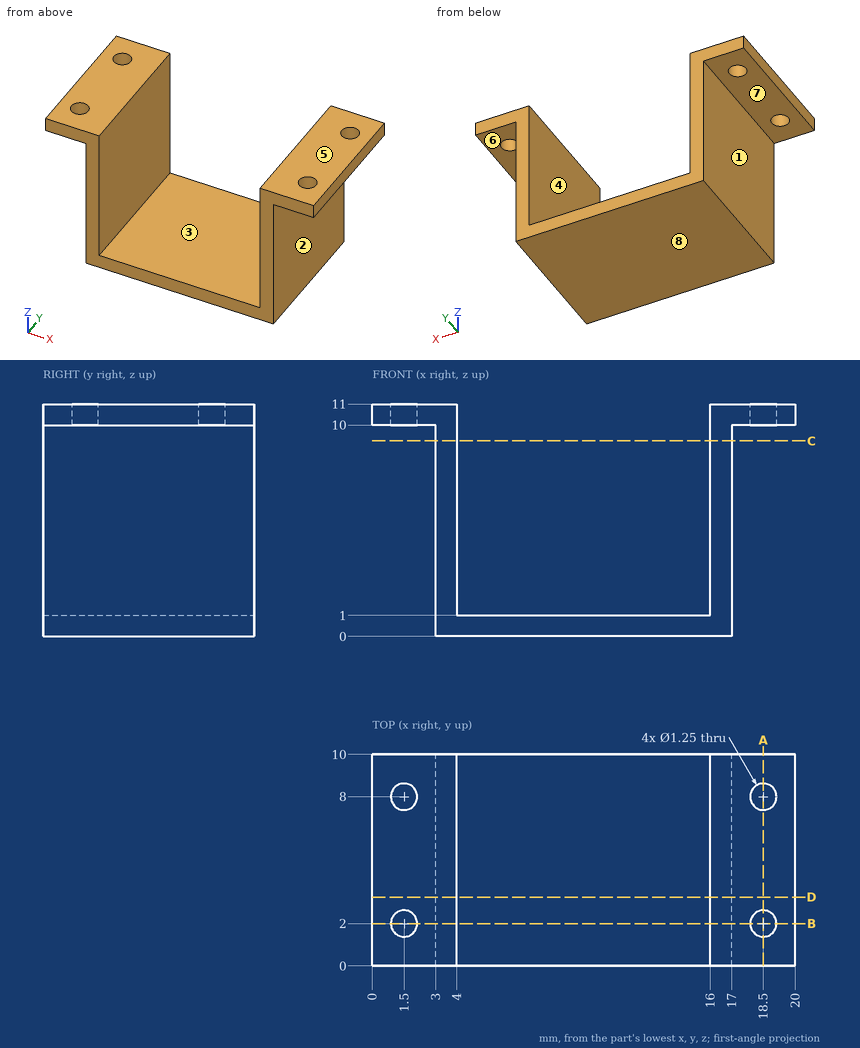
Can you work these out from the drawing? Everything is in mm from the part's minimum corner. A direction names the side the tool comes from. Coordinates: 2 decimals unless noted, no trailing zeros. Order: outer loops, then holes, each group sorted by start corner. A loop starts at its lowest first (then second) coordinate and runs counter-clockwise, first axis right, second up. Notation, with made-up numbers: M -27,54 L 30,54 A15 cw 30,61 Z; hole C 79.5,21 d3. An arc over 180 degrees is marked long. Answer as CSV lines item,"result". Start each with the question number.
1. For pin 1 (1.1 mm diameter, centred on x = 18.5, y = 2, fed in from -Z); pin 2 (3.5 mm diameter, centred on x = 1, y = 6, fed in from -Z); pin 3 (4 mm diameter, centred on x = 5, z = 6.5, fed in from +Y); pin 4 (3 mm diameter, centred on y = 3.5, z = 6, fed in from +X), each with a flat end and sliding along its axis, tell me the tip position at first contact or that it passes through.
2. I want a section at C-C, the plane z = 9.25. Write out the boundary of the cut face in (x, y), and give its area (3 significant figures).
3. I want a section at A-A, the plane x = 18.5. Write out the boundary of the cut face in (y, z) (3 decimals), and give its area (3 significant figures).
4. On a 3-axis mill with a long thin cutter (end or side, diameter ignored), from which of +Z, -Z, +X, -X, +Y, -Y can I reach the whole of each face in a straight line? I mean the marked faces 4, 5, 6, 7 and 8. Say none if no direction works.
5. We'd pull the mould along X, two halves only. Please class the marked faces 1, 2 and 3: released by +X, released by -X, zero draft, split by the parting line, or undercut.
6. I need wall thicknesses on line 1 (Y direction, x = 1.5, z = 10.65) (3 decimals); line 2 (X direction, y = 8.5, z = 7.25); line 3 (Z direction, x = 11, y = 2). Which ranges of each line are inside material? Lowest first, please. Write a range as [from, to].
7. I want a section at B-B, the plane y = 2. Write out the boundary of the cut face in (x, z) (3 decimals), and give its area (3 significant figures).
8. I want a section at D-D, the plane y = 3.25. Write out the boundary of the cut face in (x, z), and give its area (3 significant figures).
Recorded:
1,pin 1,"passes through"
1,pin 2,"stops at z = 10"
1,pin 3,"stops at y = 10"
1,pin 4,"stops at x = 17"
2,outline,"M 3,0 L 4,0 L 4,10 L 3,10 Z; M 16,0 L 17,0 L 17,10 L 16,10 Z"
2,area,"20.0 mm2"
3,outline,"M 0,10 L 1.375,10 L 1.375,11 L 0,11 Z; M 2.625,10 L 7.375,10 L 7.375,11 L 2.625,11 Z; M 8.625,10 L 10,10 L 10,11 L 8.625,11 Z"
3,area,"7.50 mm2"
4,face 4,"+Z, +Y, -Y"
4,face 5,"+Z, +X, -X, +Y, -Y"
4,face 6,"-Z, +X, +Y, -Y"
4,face 7,"-Z, -X, +Y, -Y"
4,face 8,"-Z, +X, -X, +Y, -Y"
5,face 1,"released by -X"
5,face 2,"released by +X"
5,face 3,"undercut"
6,line 1,"y = [0, 1.375], [2.625, 7.375], [8.625, 10]"
6,line 2,"x = [3, 4], [16, 17]"
6,line 3,"z = [0, 1]"
7,outline,"M 0,10 L 0.875,10 L 0.875,11 L 0,11 Z; M 2.125,10 L 3,10 L 3,0 L 17,0 L 17,10 L 17.875,10 L 17.875,11 L 16,11 L 16,1 L 4,1 L 4,11 L 2.125,11 Z; M 19.125,10 L 20,10 L 20,11 L 19.125,11 Z"
7,area,"37.5 mm2"
8,outline,"M 0,10 L 3,10 L 3,0 L 17,0 L 17,10 L 20,10 L 20,11 L 16,11 L 16,1 L 4,1 L 4,11 L 0,11 Z"
8,area,"40.0 mm2"
